Verification items for this drawing (mm, ordinates from the low corner). Give positions to 0.01 mm unless a question says otherwise; leave off trailing zeros. Order: outer loops, then holes, each group sorted by start corner. A loop starts at its lowest first (then second) coordinate and runs counter-clockwise, first axis right, second up. Notation, with made-up numbers: M 12.25,61 L 58.25,61 A24 ccw 58.25,97 Z; hole C -8,25.25 d10. An arc over 180 degrees is marked long. Return JSON: item names as keys, results as strings. Group by question number.
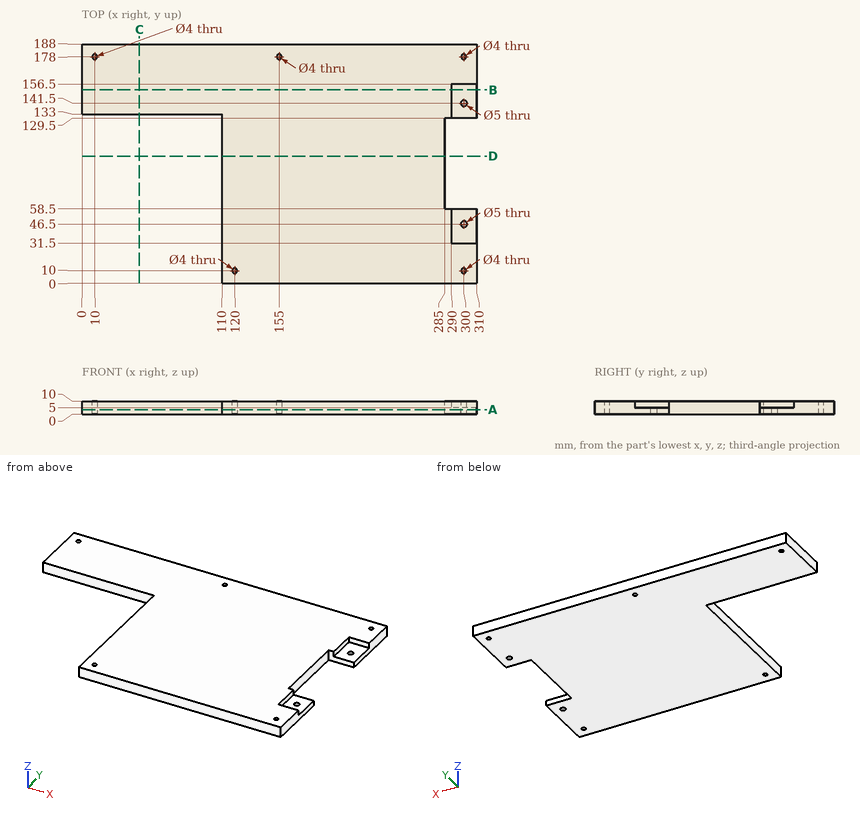
1) Sectioned sample at B-B on y = 152. Record the boundary of the cut face in (x, z).
2) Sectioned sample at D-D on y = 100. Record the boundary of the cut face in (x, z).
3) Material ranges on line 1 along X through (y, z) = (178, 3.25); line 2 along Y through (x, z) = (300, 4.5); line 3 along X through (y, z) = (141.5, 1.1), recorded low to high.
4) Sectioned sample at C-C on x = 45. Record the boundary of the cut face in (y, z).
5) Sectioned sample at A-A on z = 3.5. Record the boundary of the cut face in (x, y), then the cut area to 3 significant figures.
6) Depth check by flat-ended pin: P1, Ø6, axis at x = 299, y = 45.5, coming from the +Z side; P2, Ø4, axis at y = 143.5, z = 8.5, coming from the +X side; P3, Ø1.5, axis at x = 77.5, z = 8.5, coming from the -Y side. Enter the tip coordinate at first touch or a pass-through.
Reply:
{
 "1": {"outline": "M 0,0 L 310,0 L 310,5 L 290,5 L 290,10 L 0,10 Z"},
 "2": {"outline": "M 110,0 L 285,0 L 285,10 L 110,10 Z"},
 "3": {"line 1": "0 to 8, 12 to 153, 157 to 298, 302 to 310", "line 2": "0 to 8, 12 to 44, 49 to 58.5, 129.5 to 139, 144 to 176, 180 to 188", "line 3": "0 to 297.5, 302.5 to 310"},
 "4": {"outline": "M 133,0 L 188,0 L 188,10 L 133,10 Z"},
 "5": {"outline": "M 0,133 L 110,133 L 110,0 L 310,0 L 310,58.5 L 285,58.5 L 285,129.5 L 310,129.5 L 310,188 L 0,188 Z; hole C 10,178 d4; hole C 120,10 d4; hole C 155,178 d4; hole C 300,46.5 d5; hole C 300,141.5 d5; hole C 300,10 d4; hole C 300,178 d4", "area": "41,800 mm^2"},
 "6": {"P1": "z = 5", "P2": "x = 290", "P3": "y = 133"}
}
